```python
from build123d import *

# Parameters (mm, degrees)
SKETCH1_W           = 69.85
SKETCH1_H           = 6.35
BOSS_EXTRUDE1_DEPTH = 41.275
SHELL1_T            = -2.54
SKETCH2_W           = 12.7
SKETCH2_H           = 12.7
BOSS_EXTRUDE2_DEPTH = 3.175


with BuildPart() as part:
    # Sketch1 → Boss-Extrude1 (new, symmetric)
    with BuildSketch(Plane.XY):
        with Locations((0, 3.175)):
            Rectangle(SKETCH1_W, SKETCH1_H)
    extrude(amount=BOSS_EXTRUDE1_DEPTH, both=True)

    # Shell1
    shell1_openings = [part.faces().sort_by_distance(p)[0] for p in [
        (0, 0, 0),
    ]]
    offset(amount=SHELL1_T, openings=shell1_openings, kind=Kind.INTERSECTION)

    # Sketch2 → Boss-Extrude2 (add, symmetric)
    with BuildSketch(Plane.XY):
        with Locations((0, 12.7)):
            Rectangle(SKETCH2_W, SKETCH2_H)
    extrude(amount=BOSS_EXTRUDE2_DEPTH, both=True)


solid = part.part
```
Here's how the part is built. I have some questions about the finished solid (model axes, mm). A direction names the side the tool comes from. Coordinates: 2 decimals unless noted, no trailing zeros. Write each loop counter-clockwise with the first axis right and the second up, starting at its lowest first coordinate (ties: lowest second). Pieces come first, ordered by that corner, then holes. Notation, with made-up numbers: (-6, 32) - (-2, 32) arc R21 cw to (-2, 61) - close; hole circle Ø8 at (12.25, 74). An arc over 180 degrees is marked (long way). One line per item, written item: value.
1) I'm going to push flat-ended pins straight in: P1, Ø10, axis at x = 2.5, y = 15, coming from the -Z side (3 decimals); P2, Ø8, axis at x = -3.5, z = -8, coming from the -Y side; P3, Ø3, axis at x = 9.5, y = 12, coming from the -Z side; P4, Ø3, axis at x = -22.5, z = 13.5, coming from the +Y side. Where does each tip first touch, or does it pass through?
Model answer:
P1: stops at z = -3.175
P2: stops at y = 3.81
P3: passes through
P4: stops at y = 6.35
2) Suppose I cut it at C-C on z = 32.5. Write out the boundary of the cut face in (x, y) (3 decimals).
Model answer:
outline: (-34.925, 0) - (-32.385, 0) - (-32.385, 3.81) - (32.385, 3.81) - (32.385, 0) - (34.925, 0) - (34.925, 6.35) - (-34.925, 6.35) - close
3) Suppose I cut it at D-D on y = 16. Write out the boundary of the cut face in (x, z) (3 decimals), and give its area (3 significant figures).
Model answer:
outline: (-6.35, -3.175) - (6.35, -3.175) - (6.35, 3.175) - (-6.35, 3.175) - close
area: 80.6 mm²
4) I need wall thicknesses on line 1 along Z through (x, y) = (-32, 3) (3 decimals); line 2 along X through (y, z) = (2.5, 10) (3 decimals); line 3 along Y through (x, z) = (6, -29). Which ranges of each line are inside material? Lowest first, please.
Model answer:
line 1: z = -41.275 to -38.735, 38.735 to 41.275
line 2: x = -34.925 to -32.385, 32.385 to 34.925
line 3: y = 3.81 to 6.35
5) Suppose I cut it at B-B on y = 1.75. Write out the boundary of the cut face in (x, z) (3 decimals).
Model answer:
outline: (-34.925, -41.275) - (34.925, -41.275) - (34.925, 41.275) - (-34.925, 41.275) - close; hole (-32.385, -38.735) - (32.385, -38.735) - (32.385, 38.735) - (-32.385, 38.735) - close
6) We'd pull the mould along X, two halves only. Please class faces 1 (the flat face through (0, 3, -41.275)), 2 (the flat face through (-34.925, 3, 1)), 3 (the flat face through (6.35, 13, 0)), 4 (the flat face through (0, 2, -38.735)): pulls with the +X half, pulls with the -X half, needs draft (parallel to the pull), parting line crosses it, or undercut.
Model answer:
face 1: needs draft
face 2: pulls with the -X half
face 3: pulls with the +X half
face 4: undercut
7) On a 3-axis mill with a long thin cutter (end or side, diameter ignored), from which of +Z, -Z, +X, -X, +Y, -Y can I reach the whole of each face in a straight line? I mean faces 5 (the flat face through (0, 13, -3.175)), 6 (the flat face through (0, 13, 3.175)), 7 (the flat face through (-6.35, 13, 0)), 8 (the flat face through (0, 2, 38.735)). Say none if no direction works.
Model answer:
face 5: -Z, +X, -X, +Y
face 6: +Z, +X, -X, +Y
face 7: +Z, -Z, -X, +Y
face 8: -Y
8) Suppose I cut it at A-A on x = 3. Write out the boundary of the cut face in (y, z) (3 decimals), and give its area (3 significant figures).
Model answer:
outline: (0, -41.275) - (6.35, -41.275) - (6.35, -3.175) - (19.05, -3.175) - (19.05, 3.175) - (6.35, 3.175) - (6.35, 41.275) - (0, 41.275) - (0, 38.735) - (3.81, 38.735) - (3.81, -38.735) - (0, -38.735) - close
area: 310 mm²
